```python
from build123d import *

# Parameters (mm, degrees)
SKETCH_W        = 120
SKETCH_H        = 50
PAD_DEPTH       = 3
SKETCH001_R     = 4
POCKET_DEPTH    = 5
SKETCH002_W     = 120
SKETCH002_H     = 50
SKETCH002_W_2   = 116
SKETCH002_H_2   = 46
PAD001_DEPTH    = 30
SKETCH003_R     = 1.6
POCKET001_DEPTH = 5
SKETCH004_R     = 4
PAD002_DEPTH    = 28
SKETCH005_R     = 1.4
POCKET002_DEPTH = 26
CHAMFER_SIZE    = 0.5
CHAMFER001_SIZE = 1


with BuildPart() as part:
    # Sketch → Pad (new body)
    with BuildSketch(Plane.XY):
        Rectangle(SKETCH_W, SKETCH_H)
    extrude(amount=PAD_DEPTH)

    # Sketch001 (on Face6 of Pad) → Pocket (cut)
    with BuildSketch(Plane.XY.offset(3)):
        with Locations((10, 19)):
            Circle(SKETCH001_R)
        with Locations((22, 19)):
            Circle(SKETCH001_R)
        with Locations((34, 19)):
            Circle(SKETCH001_R)
        with Locations((46, 19)):
            Circle(SKETCH001_R)
    extrude(amount=-POCKET_DEPTH, mode=Mode.SUBTRACT)

    # Sketch002 (on Face5 of Pocket) → Pad001 (join)
    with BuildSketch(Plane.XY.offset(3)):
        Rectangle(SKETCH002_W, SKETCH002_H)
        Rectangle(SKETCH002_W_2, SKETCH002_H_2, mode=Mode.SUBTRACT)
    extrude(amount=PAD001_DEPTH)

    # Sketch003 (on Face4 of Pad001) → Pocket001 (cut)
    with BuildSketch(Plane(origin=(0, 0, 0), x_dir=(1, 0, 0), z_dir=(0, 0, -1))):
        with Locations((-20, -12.5)):
            Circle(SKETCH003_R)
        with Locations((0, -12.5)):
            Circle(SKETCH003_R)
        with Locations((20, -12.5)):
            Circle(SKETCH003_R)
    extrude(amount=-POCKET001_DEPTH, mode=Mode.SUBTRACT)

    # Sketch004 (on Face18 of Pocket001) → Pad002 (join)
    with BuildSketch(Plane.XY.offset(3)):
        with Locations((-56, 21)):
            Circle(SKETCH004_R)
        with Locations((-56, -21)):
            Circle(SKETCH004_R)
        with Locations((56, 21)):
            Circle(SKETCH004_R)
        with Locations((56, -21)):
            Circle(SKETCH004_R)
    extrude(amount=PAD002_DEPTH)

    # Sketch005 (on Face29 of Pad002) → Pocket002 (cut)
    with BuildSketch(Plane.XY.offset(31)):
        with Locations((-56, 21)):
            Circle(SKETCH005_R)
        with Locations((56, 21)):
            Circle(SKETCH005_R)
        with Locations((56, -21)):
            Circle(SKETCH005_R)
        with Locations((-56, -21)):
            Circle(SKETCH005_R)
    extrude(amount=-POCKET002_DEPTH, mode=Mode.SUBTRACT)

    # Chamfer
    chamfer_edges = [part.edges().sort_by_distance(p)[0] for p in [
        (54.6, 21, 31),
        (54.6, -21, 31),
        (-57.4, -21, 31),
        (-57.4, 21, 31),
    ]]
    chamfer(chamfer_edges, length=CHAMFER_SIZE)

    # Chamfer001
    chamfer001_edges = [part.edges().sort_by_distance(p)[0] for p in [
        (0, 25, 0),
        (-60, 0, 0),
        (0, -25, 0),
        (60, 0, 0),
    ]]
    chamfer(chamfer001_edges, length=CHAMFER001_SIZE)


solid = part.part
```
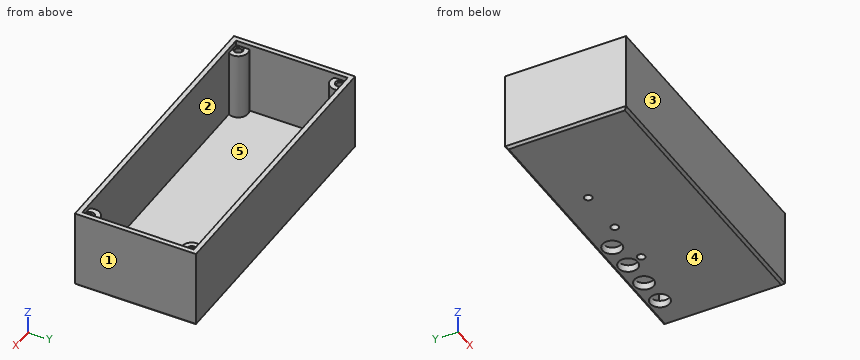
The listing builds one solid part. Answer for the finished solid, in the listing's coordinates (mm). Face numbers are marked on the shaded views. A direction names the side the tool comes from. Give positions to 0.01 mm unless a question says otherwise; leave off trailing zeros. Write each loop counter-clockwise with the first axis right and the second up, starting at its lowest first coordinate (ties: lowest second). Pieces come first, ordered by that corner, then holes. Notation, with made-up numbers: (-27.75, 24) -> (-17.75, 24) arc R24 cw to (-17.75, 53) -> close; hole circle Ø11 at (-21.75, 27). An arc over 180 degrees is marked (long way). Write item = value, one per line. Start each with the question number.
1) Which of the six approach directions +Z, -Z, +X, -X, +Y, -Y give full straight-line access (tool end or side, diameter ignored) to the marked faces 4 and 5?
2) Straight lines are drawn through the part: line 1 along Y through (x, z) = (-56, 23.25); line 2 along Y through (x, z) = (0, 1.5); line 3 along X through (y, z) = (-5.5, 28). For each, find the intervals that lie inside material, in ascending order.
3) The part is cut by section C-C, the plane y = 8. Determine the outline of the cut face in (x, z).
4) The part is cut by section A-A, the plane x = 0. Determine the outline of the cut face in (y, z).
5) The part is cut by section D-D, the plane z = 18. Determine the outline of the cut face in (x, y), and give its area (3 significant figures).
6) Determine the mould class of the marked faces 1, 2 and 3 for opening direction X: +X half, -X half, draft (parallel to the pull), parting line (faces both ways), or undercut.
7) Each of these flat-tipped pins is pushed along its axis until it touches: pin 1 (6.5 mm diameter, centred on x = -54.5, y = -21, fed in from +Z); pin 2 (1.8 mm diameter, centred on x = 54, y = -20.5, fed in from +Z); pin 3 (6.5 mm diameter, centred on x = 34, y = 19, fed in from +Z); pin 4 (0.8 mm diameter, centred on x = 56, y = -20.5, fed in from +Z). Where does it stop, or does it pass through?
8) The part is cut by section B-B, the plane x = 20. Determine the outline of the cut face in (y, z).
Solutions:
q1.face_4 = -Z, +X, -X, +Y, -Y
q1.face_5 = +Z
q2.line_1 = -25 to -22.4, -19.6 to -17, 17 to 19.6, 22.4 to 25
q2.line_2 = -25 to 10.9, 14.1 to 25
q2.line_3 = -60 to -58, 58 to 60
q3.outline = (-60, 1) -> (-59, 0) -> (59, 0) -> (60, 1) -> (60, 33) -> (58, 33) -> (58, 3) -> (-58, 3) -> (-58, 33) -> (-60, 33) -> close
q4.outline = (-25, 1) -> (-24, 0) -> (10.9, 0) -> (10.9, 3) -> (-23, 3) -> (-23, 33) -> (-25, 33) -> close; (14.1, 0) -> (24, 0) -> (25, 1) -> (25, 33) -> (23, 33) -> (23, 3) -> (14.1, 3) -> close
q5.outline = (-60, -25) -> (60, -25) -> (60, 25) -> (-60, 25) -> close; hole (-58, -17.54) arc R4 cw to (-52.54, -23) -> (52.54, -23) arc R4 cw to (58, -17.54) -> (58, 17.54) arc R4 cw to (52.54, 23) -> (-52.54, 23) arc R4 cw to (-58, 17.54) -> close; hole circle Ø2.8 at (-56, -21); hole circle Ø2.8 at (-56, 21); hole circle Ø2.8 at (56, -21); hole circle Ø2.8 at (56, 21)
q5.area = 767 mm²
q6.face_1 = +X half
q6.face_2 = undercut
q6.face_3 = draft
q7.pin_1 = 33
q7.pin_2 = 31
q7.pin_3 = through
q7.pin_4 = 5
q8.outline = (-25, 1) -> (-24, 0) -> (10.9, 0) -> (10.9, 3) -> (-23, 3) -> (-23, 33) -> (-25, 33) -> close; (14.1, 0) -> (15.54, 0) -> (15.54, 3) -> (14.1, 3) -> close; (22.46, 0) -> (24, 0) -> (25, 1) -> (25, 33) -> (23, 33) -> (23, 3) -> (22.46, 3) -> close
